Design review of the part built by this model. Coordinates are the model's own, in mm. Round coordinates to 2 decimals unless told otherwise and drop trailing zeros. Write each loop counter-clockwise with the first axis right and the second up, starting at its lowest first coordinate (ties: lowest second). Pieces come first, ordered by that corner, then holes. Notation, with made-up numbers: (6.25, 55) -> (18.25, 55) arc R20 ccw to (18.25, 91) -> close; hole circle Ø6 at (46, 88). An arc over 180 degrees is marked (long way). Write item = value, one per line. Start each with the question number.
Item 1: Add section B-B, the plane z = -20. State the section outline as (x, y) points.
Item 2: Add section A-A, the plane x = 33. State the section outline as (y, z) points.
Item 3: Add section C-C, the plane y = 13.5. State the section outline as (x, z) points.
Item 4: For pin 1 Ø3 at (x, z) = (138.89, -16.35) entering from +Y, flat-tipped, find the tip position at first contact; note if it passes through.
Item 5: Mouldability with a two-part tool opening along X and no side actions: class faces 1 (the flat face through (0, 9, -17)), 2 (the cylindrical face through (140.886, 8.874, -16.438)), 3 (the flat face through (74, 9, 0)) as released by +X, released by -X, zero draft, split by the parting line, or undercut.
Item 6: To check wall thickness, follow L1, parallel to X at y = 13.25, z = -16; L2, parallel to X at y = 8, z = -16.5; L3, parallel to Z at x = 33, y = 9.25. State the ranges of each line that lie inside material, in increasing order.
Autodesk Inventor part; units mm, degrees
ref_plane "YZ Plane" through (0, 0, 0) normal (1, 0, 0) x (0, 1, 0)
ref_plane "XZ Plane" through (0, 0, 0) normal (0, 1, 0) x (-1, 0, 0)
ref_plane "XY Plane" through (0, 0, 0) normal (0, 0, 1) x (1, 0, 0)
sketch "Sketch1" plane through (0, 0, 0) normal (0, 1, 0) x (-1, 0, 0)
  line L0 (0, 0) -> (-150, 0)
  line L1 (-150, 0) -> (-150, -32.7)
  line L2 (-150, -32.7) -> (0, -32.7)
  line L3 (0, -32.7) -> (0, 0)
  circle A0 centre (-33, -16.35) radius 5.5563
  circle A1 centre (-138.8875, -16.35) radius 2
  point P0 (0, -16.35)
  point P1 (-150, -16.35)
  dimension "d0" = 150
  dimension "d1" = 32.7
  dimension "d2" = 33
  dimension "d3" = 11.1125
  dimension "d4" = 11.1125
  dimension "Diametro_eje_pequeño" = 4
extrude "Extrusion1" add sketch "Sketch1" along normal blind 18
fillet "Fillet1" radius 3 4 edges at (0, 9, 0) (150, 9, 0) (150, 9, -32.7) (0, 9, -32.7)
equation "\"d1\" = ancho"
equation "\"d2\" = separacion_grande"
equation "\"d3\" = diametro_interno"
equation "\"d4\" = d3"
equation "\"Diametro_eje_pequeño\" = Diametro_eje_pequeño_1"
properties part number "Transmisor_grande" material "Aluminum 6061"
Result set:
q1.outline = (0, 0) -> (28.81, 0) -> (28.81, 18) -> (0, 18) -> close; (37.19, 0) -> (150, 0) -> (150, 18) -> (37.19, 18) -> close
q2.outline = (0, -32.7) -> (18, -32.7) -> (18, -21.91) -> (0, -21.91) -> close; (0, -10.79) -> (18, -10.79) -> (18, 0) -> (0, 0) -> close
q3.outline = (0, -29.7) arc R3 ccw to (3, -32.7) -> (147, -32.7) arc R3 ccw to (150, -29.7) -> (150, -3) arc R3 ccw to (147, 0) -> (3, 0) arc R3 ccw to (0, -3) -> close; hole circle Ø11.11 at (33, -16.35); hole circle Ø4 at (138.89, -16.35)
q4.pin_1 = through
q5.face_1 = released by -X
q5.face_2 = undercut
q5.face_3 = zero draft
q6.L1 = 0 to 27.45, 38.55 to 136.92, 140.86 to 150
q6.L2 = 0 to 27.45, 38.55 to 136.89, 140.88 to 150
q6.L3 = -32.7 to -21.91, -10.79 to 0
